Source: CAD feature listing. Evaluate the final solid. Frame: model axes, mm. Face numbers are marked on the shaded views. A direction names the side the tool comes from. Give positions to 0.01 mm unless a question says otherwise; leave off trailing zeros. Loops run counter-clockwise (first coordinate to the right, second up) from the corner with the lowest first, then second, coordinate; pieces in that order, holes last. Notation, with made-up numbers: (-8, 18.25) -> (45, 18.25) arc R15 ccw to (45, 30.25) -> close; hole circle Ø8 at (-36, 9.25). An arc over 180 degrees is marked (long way). Return JSON: item names as keys, results as strings. Group by question number.
(1) Ray query, line 1 (Z direction, x = 4.5, y = -6); line 2 (Y direction, x = 5, z = 28.5). Return the intervals inside material, ascending. Write a range as from..to.
(2) Access query for the marked faces 1 and 2. Directions: +Z, -Z, +X, -X, +Y, -Y. A direction counts if a zero-diameter tool reaches every point of the face in a straight line with its end or side. Return the directions, or none.
(3) Cut plane C-C on x = -3.25. Return loops of the section in (y, z), then the cut area to 3 significant figures.
(4) Cut plane B-B on y = 1.25. Return loops of the section in (x, z), then the cut area to 3 significant figures.
(5) Pin query (flat end, axial travel): pin 1 (8 mm diameter, centred on x = -1, y = 3.5, fed in from -Z); pin 2 (1.6 mm diameter, centred on y = -9.5, z = -28, fed in from +X); pin 3 (2 mm diameter, centred on y = -9, z = 27, fed in from +X). Return the tip coordinate at first contact, or that it passes through.
(6) Cut plane A-A on x = 0. Return loops of the section in (y, z).
```python
from build123d import *

# Parameters (mm, degrees)
SKETCH_1_W      = 25
SKETCH_1_H      = 20
EXTRUDE_1_DEPTH = 22
EXTRUDE_2_DEPTH = 2
FILLET_1_R      = 2


with BuildPart() as part:
    # 草图1 → 凸台-拉伸1 (new, symmetric)
    with BuildSketch(Plane.XY):
        Rectangle(SKETCH_1_W, SKETCH_1_H)
    extrude(amount=EXTRUDE_1_DEPTH, both=True)

    # 草图2 → 凸台-拉伸2 (add)
    with BuildSketch(Plane.XZ.offset(10)):
        with BuildLine():
            Line((-8.5, -22), (-6.161301565, -29.589004522))
            ThreePointArc((-6.161301565, -29.589004522), (-3.952177176, -30.977701081), (-2.25, -29))
            Line((-2.25, -29), (-2.25, -26))
            ThreePointArc((-2.25, -26), (0, -23.75), (2.25, -26))
            Line((2.25, -26), (2.25, -29))
            ThreePointArc((2.25, -29), (3.952177176, -30.977701081), (6.161301565, -29.589004522))
            Line((6.161301565, -29.589004522), (8.5, -22))
            Line((8.5, -22), (-8.5, -22))
        make_face()
        with BuildLine():
            Line((-8.5, 22), (8.5, 22))
            Line((8.5, 22), (6.161301565, 29.589004522))
            ThreePointArc((6.161301565, 29.589004522), (3.952177176, 30.977701081), (2.25, 29))
            Line((2.25, 29), (2.25, 26))
            ThreePointArc((2.25, 26), (0, 23.75), (-2.25, 26))
            Line((-2.25, 26), (-2.25, 29))
            ThreePointArc((-2.25, 29), (-3.952177176, 30.977701081), (-6.161301565, 29.589004522))
            Line((-6.161301565, 29.589004522), (-8.5, 22))
        make_face()
    extrude(amount=-EXTRUDE_2_DEPTH)

    # 圆角1
    fillet_1_edges = [part.edges().sort_by_distance(p)[0] for p in [
        (-12.5, 10, 0),
        (12.5, 10, 0),
    ]]
    fillet(fillet_1_edges, radius=FILLET_1_R)


solid = part.part
```
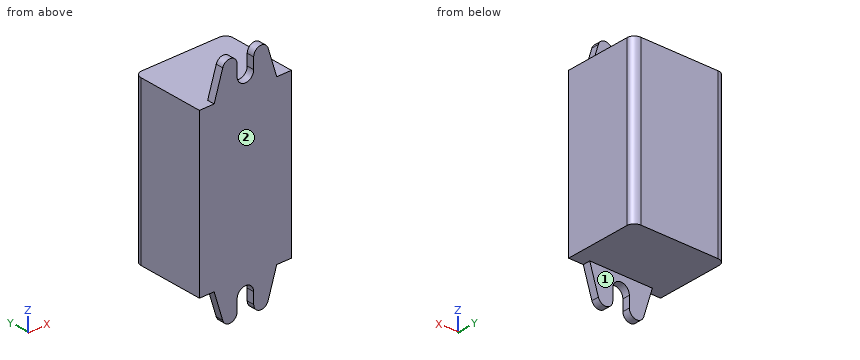
Answers:
{
 "1": {"line 1": "-22..22", "line 2": "-10..-8"},
 "2": {"face 1": "-Z, +X, -X, +Y", "face 2": "+Z, -Z, +X, -X, -Y"},
 "3": {"outline": "(-10, -30.73) -> (-8, -30.73) -> (-8, -22) -> (10, -22) -> (10, 22) -> (-8, 22) -> (-8, 30.73) -> (-10, 30.73) -> close", "area": "915 mm²"},
 "4": {"outline": "(-12.5, -22) -> (12.5, -22) -> (12.5, 22) -> (-12.5, 22) -> close", "area": "1,100 mm²"},
 "5": {"pin 1": "z = -22", "pin 2": "x = 6.9", "pin 3": "x = 7.27"},
 "6": {"outline": "(-10, -23.75) -> (-8, -23.75) -> (-8, -22) -> (10, -22) -> (10, 22) -> (-8, 22) -> (-8, 23.75) -> (-10, 23.75) -> close"}
}
